from build123d import *

# Parameters (mm, degrees)
BOSS_EXTRUDE2_DEPTH      = 8
BOSS_EXTRUDE2_DEPTH_BACK = 1
SKETCH1_W                = 66
SKETCH1_H                = 19
SKETCH3_R                = 2.75
BOSS_EXTRUDE3_DEPTH      = 13.75
SKETCH4_W                = 4.5
SKETCH4_H                = 6.5
BOSS_EXTRUDE4_DEPTH      = 15
BOSS_EXTRUDE5_DEPTH      = 8.5
SKETCH8_W                = 9
SKETCH8_H                = 6.5
BOSS_EXTRUDE6_DEPTH      = 6
SKETCH9_W                = 15.5
SKETCH9_H                = 6.5
BOSS_EXTRUDE7_DEPTH      = 21
BOSS_EXTRUDE8_DEPTH      = 8.5
CUT_EXTRUDE2_START       = -8.5
SKETCH12_R               = 3.5
CUT_EXTRUDE2_DEPTH       = 8.5
FILLET1_R                = 10
SKETCH14_W               = 15
SKETCH14_H               = 9
BOSS_EXTRUDE10_DEPTH     = 65
CUT_EXTRUDE3_REACH       = 91.135
SKETCH15_R               = 2.5


with BuildPart() as part:
    # Sketch1 → Boss-Extrude2 (new, two sides: drawn at the far end of the back side and taken through both)
    with BuildSketch(Plane(origin=(0, 0, 0), x_dir=(1, 0, 0), z_dir=(0, 1, 0)).offset(-BOSS_EXTRUDE2_DEPTH_BACK)):
        with Locations((22, 18)):
            Rectangle(SKETCH1_W, SKETCH1_H)
    extrude(amount=BOSS_EXTRUDE2_DEPTH + BOSS_EXTRUDE2_DEPTH_BACK)

    # Sketch3 → Boss-Extrude3 (add)
    with BuildSketch(Plane(origin=(0, 0, -27.5), x_dir=(-1, 0, 0), z_dir=(0, 0, -1))):
        with Locations((-37.5, 3.5)):
            Circle(SKETCH3_R)
        with Locations((-17.5, 3.5)):
            Circle(SKETCH3_R)
    extrude(amount=BOSS_EXTRUDE3_DEPTH)

    # Sketch4 → Boss-Extrude4 (add)
    with BuildSketch(Plane(origin=(0, 8, 0), x_dir=(1, 0, 0), z_dir=(0, 1, 0))):
        with Locations((25.25, 20.75)):
            Rectangle(SKETCH4_W, SKETCH4_H)
        with Locations((29.75, 20.75)):
            Rectangle(SKETCH4_W, SKETCH4_H)
    extrude(amount=BOSS_EXTRUDE4_DEPTH)

    # Sketch5 → Boss-Extrude5 (add)
    with BuildSketch(Plane(origin=(0, 0, -24), x_dir=(-1, 0, 0), z_dir=(0, 0, -1))):
        with BuildLine():
            ThreePointArc((-25.636419782, 13.037388184), (-24.436298745, 14.307742745), (-24, 16))
            ThreePointArc((-24, 16), (-29.974873734, 18.474873734), (-27.5, 12.5))
            ThreePointArc((-27.5, 12.5), (-26.685966178, 12.595980474), (-25.916578842, 12.878657751))
            ThreePointArc((-25.916578842, 12.878657751), (-25.85405917, 13.094916041), (-25.636419782, 13.037388184))
        make_face()
    extrude(amount=BOSS_EXTRUDE5_DEPTH)

    # Sketch8 → Boss-Extrude6 (add)
    with BuildSketch(Plane(origin=(0, 23, 0), x_dir=(1, 0, 0), z_dir=(0, 1, 0))):
        with Locations((27.5, 20.75)):
            Rectangle(SKETCH8_W, SKETCH8_H)
    extrude(amount=BOSS_EXTRUDE6_DEPTH)

    # Sketch9 → Boss-Extrude7 (add)
    with BuildSketch(Plane(origin=(0, 8, 0), x_dir=(1, 0, 0), z_dir=(0, 1, 0))):
        with Locations((15.25, 20.75)):
            Rectangle(SKETCH9_W, SKETCH9_H)
        with Locations((39.75, 20.75)):
            Rectangle(SKETCH9_W, SKETCH9_H)
    extrude(amount=BOSS_EXTRUDE7_DEPTH)

    # Sketch10 → Boss-Extrude8 (add)
    with BuildSketch(Plane(origin=(0, 0, -24), x_dir=(-1, 0, 0), z_dir=(0, 0, -1))):
        with BuildLine():
            Line((-21, 17), (-17.5, 17))
            Line((-17.5, 17), (-14, 17))
            ThreePointArc((-14, 17), (-17.5, 20.5), (-21, 17))
        make_face()
        with BuildLine():
            Line((-17.5, 13.5), (-17.5, 17))
            Line((-17.5, 17), (-21, 17))
            ThreePointArc((-21, 17), (-19.974873734, 14.525126266), (-17.5, 13.5))
        make_face()
        with BuildLine():
            Line((-14, 17), (-17.5, 17))
            Line((-17.5, 17), (-17.5, 13.5))
            ThreePointArc((-17.5, 13.5), (-15.025126266, 14.525126266), (-14, 17))
        make_face()
        with BuildLine():
            Line((-37.5, 17), (-34, 17))
            ThreePointArc((-34, 17), (-37.5, 20.5), (-41, 17))
            Line((-41, 17), (-37.5, 17))
        make_face()
        with BuildLine():
            ThreePointArc((-37.5, 13.5), (-35.025126266, 14.525126266), (-34, 17))
            Line((-34, 17), (-37.5, 17))
            Line((-37.5, 17), (-37.5, 13.5))
        make_face()
        with BuildLine():
            Line((-37.5, 13.5), (-37.5, 17))
            Line((-37.5, 17), (-41, 17))
            ThreePointArc((-41, 17), (-39.974873734, 14.525126266), (-37.5, 13.5))
        make_face()
    extrude(amount=BOSS_EXTRUDE8_DEPTH)

    # Sketch12 → Cut-Extrude2 (cut)
    with BuildSketch(Plane(origin=(0, 0, -32.5), x_dir=(-1, 0, 0), z_dir=(0, 0, -1)).offset(CUT_EXTRUDE2_START)):
        with Locations((-27.5, 16)):
            Circle(SKETCH12_R)
    extrude(amount=CUT_EXTRUDE2_DEPTH, mode=Mode.SUBTRACT)

    # Fillet1
    fillet1_edges = [part.edges().sort_by_distance(p)[0] for p in [
        (7.5, 29, -20.75),
        (47.5, 29, -20.75),
    ]]
    fillet(fillet1_edges, radius=FILLET1_R)

    # Sketch14 → Boss-Extrude10 (add)
    with BuildSketch(Plane.XZ.offset(1)):
        with Locations((47.5, -13)):
            Rectangle(SKETCH14_W, SKETCH14_H)
    extrude(amount=BOSS_EXTRUDE10_DEPTH)

    # Sketch15 → Cut-Extrude3 (cut, up to next)
    with BuildSketch(Plane(origin=(0, 0, -17.5), x_dir=(-1, 0, 0), z_dir=(0, 0, -1)), mode=Mode.PRIVATE) as cut_extrude3_sk1:
        with Locations((-47.5, -58.5)):
            Circle(SKETCH15_R)
    cut_extrude3_tool1 = extrude(cut_extrude3_sk1.sketch, amount=-CUT_EXTRUDE3_REACH, mode=Mode.PRIVATE) & part.part
    # Sketch15 → Cut-Extrude3 (cut, up to next)
    with BuildSketch(Plane(origin=(0, 0, -17.5), x_dir=(-1, 0, 0), z_dir=(0, 0, -1)), mode=Mode.PRIVATE) as cut_extrude3_sk2:
        with Locations((-47.5, -18.5)):
            Circle(SKETCH15_R)
    cut_extrude3_tool2 = extrude(cut_extrude3_sk2.sketch, amount=-CUT_EXTRUDE3_REACH, mode=Mode.PRIVATE) & part.part
    add(cut_extrude3_tool1.solids().sort_by_distance((47.5, -58.5, -17.5))[0], mode=Mode.SUBTRACT)
    add(cut_extrude3_tool2.solids().sort_by_distance((47.5, -18.5, -17.5))[0], mode=Mode.SUBTRACT)


solid = part.part
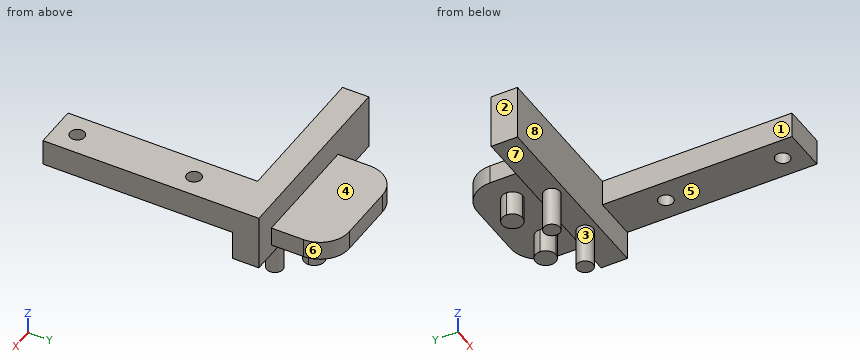
The model under review builds one solid part; all positions refer to its coordinate system, in mm. Face numbers are marked on the shaded views. A direction names the side the tool comes from. Round coordinates to 2 decimals unless told otherwise and drop trailing zeros. Loops run counter-clockwise (first coordinate to the right, second up) from the corner with the lowest first, then second, coordinate; pieces in that order, holes last. Notation, with made-up numbers: (27, 54) -> (73, 54) arc R13 ccw to (73, 66) -> close; hole circle Ø7 at (27, 21). An arc over 180 degrees is marked (long way). Return JSON: item names as keys, results as strings.
(1) Add section D-D on x = 25. Write out the cut boundary in (y, z).
Solved:
{"outline": "(-1, -27.5) -> (8, -27.5) -> (8, -24) -> (29, -24) -> (29, -17.5) -> (8, -17.5) -> (8, -8.5) -> (-1, -8.5) -> close"}
(2) For the marked faces 1, 2, 3, 4 and 5, list the 3-axis set-ups (+Z, -Z, +X, -X, +Y, -Y) from which the entire face can be reached by the end or side of a thin tool; tool diameter is ignored.
Solved:
{"face 1": "+Z, -Z, -X, -Y", "face 2": "+Z, -Z, -X, +Y, -Y", "face 3": "-Z", "face 4": "+Z, +X, -X, +Y", "face 5": "-Z, +X, -X, -Y"}
(3) Add section C-C on z = -19. Write out the cut boundary in (x, y), plus the area to 3 significant figures.
Solved:
{"outline": "(-11, -1) -> (55, -1) -> (55, 8) -> (47.5, 8) -> (47.5, 19) arc R10 ccw to (37.5, 29) -> (17.5, 29) arc R10 ccw to (7.5, 19) -> (7.5, 8) -> (-11, 8) -> close", "area": "1,390 mm2"}
(4) For line 1 (Y direction, x = 47.5, z = -11); line 2 (Y direction, x = 47, z = -10); line 3 (Z direction, x = 25.5, y = 12.5), list the stretches that pass through material, from the lowest coordinate up.
Solved:
{"line 1": "-66 to -61, -56 to -21, -16 to 8", "line 2": "-66 to -60.95, -56.05 to -20.95, -16.05 to 8", "line 3": "-24 to -17.5"}
(5) For pin 1 (5 mm diameter, centred on x = 19, z = -28, fed in from -Y); pin 2 (3 mm diameter, centred on x = 33, z = -29.5, fed in from -Y); pin 3 (16.5 mm diameter, centred on x = 44.5, y = -19, fed in from -Z); pin 4 (3 mm diameter, centred on x = 47.5, y = -18.5, fed in from -Z), all flat-tipped, find the tip position at first contact; note any pin that passes through.
Solved:
{"pin 1": "y = -1", "pin 2": "y = 15.2", "pin 3": "z = -17.5", "pin 4": "through"}
(6) Add section B-B on z = -30. Write out the cut boundary in (x, y), plus the area to 3 significant figures.
Solved:
{"outline": "circle Ø7 at (17.5, 17); circle Ø5.5 at (17.5, 3.5); circle Ø7 at (37.5, 17); circle Ø5.5 at (37.5, 3.5)", "area": "124 mm2"}
(7) Add section A-A on y = -58.5. Write out the cut boundary in (x, z).
Solved:
{"outline": "(40, -17.5) -> (45, -17.5) -> (45, -8.5) -> (40, -8.5) -> close; (50, -17.5) -> (55, -17.5) -> (55, -8.5) -> (50, -8.5) -> close"}
(8) The part is to be moulded in two halves that separate along X. For the marked faces 6, 7 and 8, say which applies: released by +X, released by -X, zero draft, split by the parting line, or undercut.
Solved:
{"face 6": "released by +X", "face 7": "undercut", "face 8": "zero draft"}
